Can you work these out from the drawing? Everything is in mm from the part's minimum corner. Round coordinates to 2 decimals unless told otherwise and drop trailing zeros. Order: outer loops, then holes, each group sorted by start corner. A loop starts at its lowest first (then second) coordinate and runs counter-clockwise, first axis right, second up. Notation, with made-up numbers: (-16.5, -14) - (5.5, -14) arc R23 cw to (5.5, 3) - close; hole circle Ø1 at (80.25, 37.5). An arc over 180 degrees is marked (long way). Write item = value, one per line.
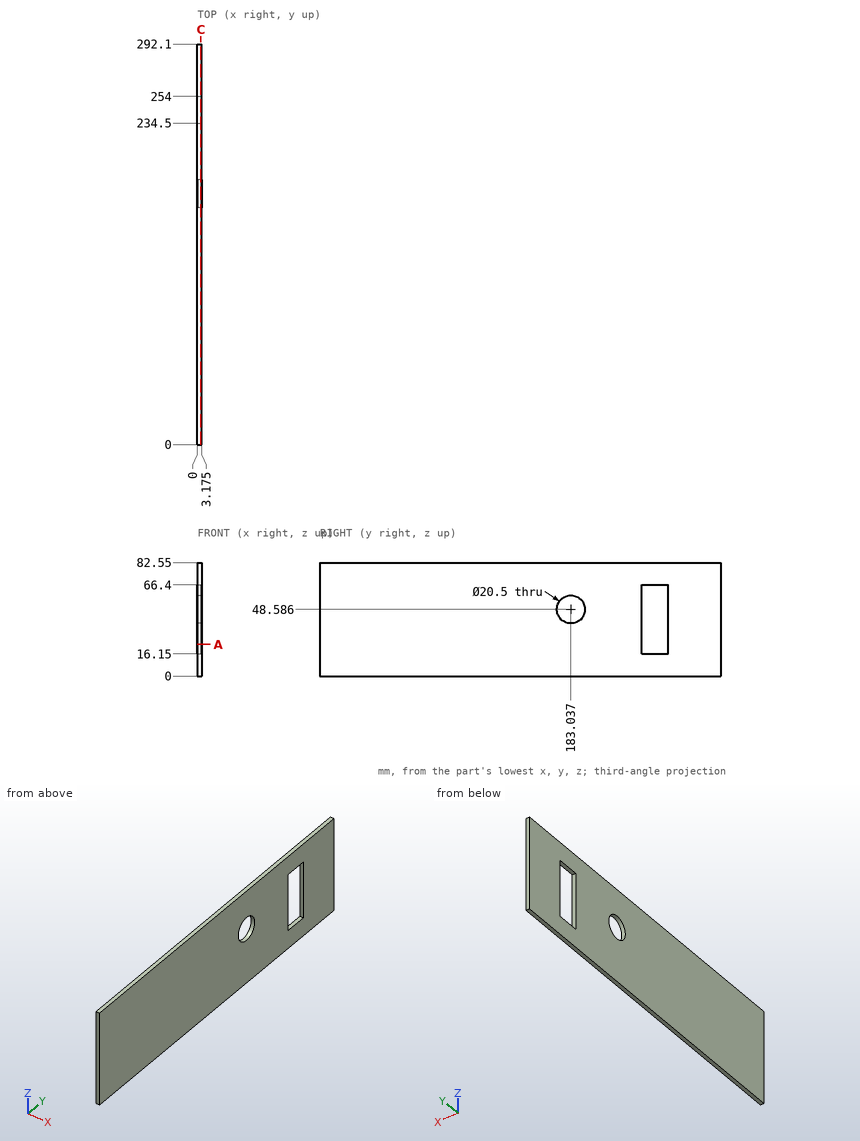
(1) If we section it at A-A (z = 23): Write out the boundary of the cut face in (x, y) (1 decimal).
Computed:
outline = (0, 0) - (3.2, 0) - (3.2, 234.5) - (0, 234.5) - close; (0, 254) - (3.2, 254) - (3.2, 292.1) - (0, 292.1) - close
(2) Will this pin go through, and if not, where does the flat tip stop? P1, Ø1, axis at x = 1.5, y = 243, coming from the -Z side.
Computed:
P1 = 0
(3) If I drill on line 1 (Y direction, x = 2, z = 49) (1 decimal); line 2 (Y direction, x = 1, z = 58) (1 decimal); line 3 (Y direction, x = 0.55, z = 31), over which ranges is the centre line in solid material (lowest first)? Write a range as from..to.
Computed:
line_1 = 0..172.8, 193.3..234.5, 254..292.1
line_2 = 0..179, 187.1..234.5, 254..292.1
line_3 = 0..234.5, 254..292.1
(4) If we section it at C-C (x = 2.55): Write out the boundary of the cut face in (y, z), plus the area to 3 significant figures.
Computed:
outline = (0, 0) - (292.1, 0) - (292.1, 82.55) - (0, 82.55) - close; hole circle Ø20.5 at (183.04, 48.59); hole (234.5, 16.15) - (254, 16.15) - (254, 66.4) - (234.5, 66.4) - close
area = 22,800 mm^2
